```python
from build123d import *

# Parameters (mm, degrees)
F0_W     = 7.5
F0_H     = 13
F0_R     = 3
F0_R_2   = 1.6
F1_DEPTH = 3
F3_DEPTH = 1
F4_DEPTH = 7.5
F5_R     = 1


with BuildPart() as f1:
    # F0 (on Top) → F1 (new body)
    with BuildSketch(Plane.XY):
        Rectangle(F0_W, F0_H)
        with Locations((0, -3)):
            Circle(F0_R, mode=Mode.SUBTRACT)
        with Locations((0, -3)):
            Circle(F0_R)
        with Locations((0, -3)):
            Circle(F0_R_2, mode=Mode.SUBTRACT)
    extrude(amount=F1_DEPTH)

    # F0 (on Top) → F3 (cut)
    with BuildSketch(Plane.XY):
        with Locations((0, -3)):
            Circle(F0_R)
        with Locations((0, -3)):
            Circle(F0_R_2, mode=Mode.SUBTRACT)
    extrude(amount=F3_DEPTH, mode=Mode.SUBTRACT)

    # F2 (on face) → F4 (join, through all)
    with BuildSketch(Plane.YZ.offset(3.75)):
        Polygon((2.7, 3), (6.5, 3), (6.5, 6), (5.7, 6), align=None)
    extrude(amount=-F4_DEPTH)

    # F5
    f5_edges = [f1.edges().sort_by_distance(p)[0] for p in [
        (3.75, -6.5, 1.5),
        (-3.75, -6.5, 1.5),
        (3.75, 6.5, 3),
        (-3.75, 6.5, 3),
    ]]
    fillet(f5_edges, radius=F5_R)


solid = f1.part
```
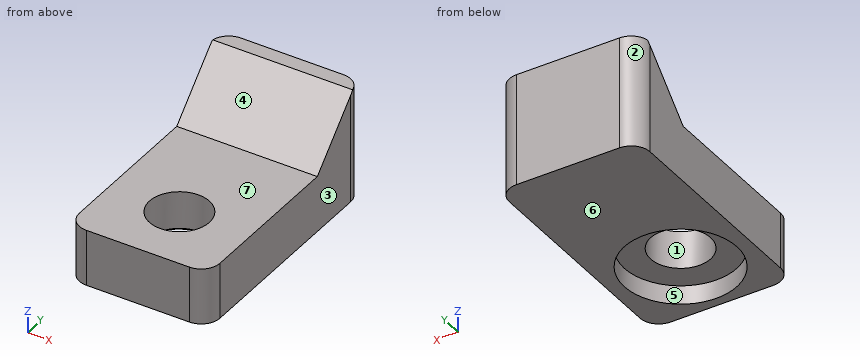
Geometry: final body of the model. Coordinates: model frame, mm. Face numbers are marked on the shaded views. A direction names the side the tool comes from. Give positions to 0.01 mm unless a question says otherwise; leave off trailing zeros. Order: outer loops, then holes, each group sorted by start corner. A loop starts at its lowest first (then second) coordinate and runs counter-clockwise, first axis right, second up. Notation, with made-up numbers: M 41,71 L 59,71 A30 ccw 59,106 Z; hole C -8,-39.5 d10. An arc over 180 degrees is marked long. Answer as CSV lines item,"result". Start each with the question number.
1) Mould query, pull axis Y, two halves, no side actions, for the marked faces 1, 2, 3 and 4. Classes: +Y half, -Y half, draft (parallel to the pull), parting line (faces both ways), or undercut.
2) Line query: line 1 (Y direction, x = 0, z = 1.55); line 2 (Y direction, x = 0, z = 0.25); line 3 (Z direction, x = -3, y = -2.5). Output: solid intervals per line, ascending. Write a range as from..to.
3) Cut plane B-B (z = 2.5). Output: boundary loops of the cut face in (x, y), then the cut area to 3 significant figures.
4) First-contact query: P1, Ø1, axis at x = 0, z = 5, coming from the -Y side; P2, Ø1.5, axis at y = -3, z = 4, coming from the -X side; P3, Ø3.5, axis at x = 0, y = -3, coming from the -Z side; P4, Ø4, axis at x = 0, y = -5, coming from the +Z side. Flat tips, straight axial feed; report the tip coordinate or a pass-through.
5) Cut plane A-A (x = 0). Output: boundary loops of the cut face in (y, z).
6) Set-up query: the marked faces 5, 6 and 7. Return all of +Z, -Z, +X, -X, +Y, -Y with unobstructed straight access to the full face (end or side cutting, diameter ignored); none if empty.
7) Cut plane C-C (y = -3). Output: boundary loops of the cut face in (x, z), then the cut area to 3 significant figures.
8) Cut plane D-D (z = 5.25). Output: boundary loops of the cut face in (x, y), then the cut area to 3 significant figures.
Findings below:
1,face 1,"undercut"
1,face 2,"+Y half"
1,face 3,"draft"
1,face 4,"-Y half"
2,line 1,"y = -6.5..-4.6, -1.4..6.5"
2,line 2,"y = -6.5..-6, 0..6.5"
2,line 3,"z = 0..3"
3,outline,"M -3.75,-5.5 A1 ccw -2.75,-6.5 L 2.75,-6.5 A1 ccw 3.75,-5.5 L 3.75,5.5 A1 ccw 2.75,6.5 L -2.75,6.5 A1 ccw -3.75,5.5 Z; hole C 0,-3 d3.2"
3,area,"88.6 mm²"
4,P1,"stops at y = 4.2"
4,P2,"passes through"
4,P3,"stops at z = 1"
4,P4,"stops at z = 3"
5,outline,"M -6.5,0 L -6,0 L -6,1 L -4.6,1 L -4.6,3 L -6.5,3 Z; M -1.4,1 L 0,1 L 0,0 L 6.5,0 L 6.5,6 L 5.7,6 L 2.7,3 L -1.4,3 Z"
6,face 5,"-Z"
6,face 6,"-Z, +X, -X, +Y, -Y"
6,face 7,"+Z, +X, -X, -Y"
7,outline,"M -3.75,0 L -3,0 L -3,1 L -1.6,1 L -1.6,3 L -3.75,3 Z; M 1.6,1 L 3,1 L 3,0 L 3.75,0 L 3.75,3 L 1.6,3 Z"
7,area,"10.1 mm²"
8,outline,"M -3.75,4.95 L 3.75,4.95 L 3.75,5.5 A1 ccw 2.75,6.5 L -2.75,6.5 A1 ccw -3.75,5.5 Z"
8,area,"11.2 mm²"
